Check sheet for the drawn part. Datum: minimum x, y, z corner. Units: mm. A direction names the side the tool comes from. Coordinates: 2 decimals unless noted, no trailing zeros. Write each loop counter-clockwise with the first axis right and the second up, starting at its lowest first coordinate (ties: lowest second). Pieces come first, ordered by that corner, then holes. Notation, with made-up numbers: (40.25, -14) -> (65.25, -14) arc R20 cw to (65.25, -10) -> close; hole circle Ø10 at (63.25, 80). An arc over 180 degrees is marked (long way). Answer in a Markdown table with one row per item.
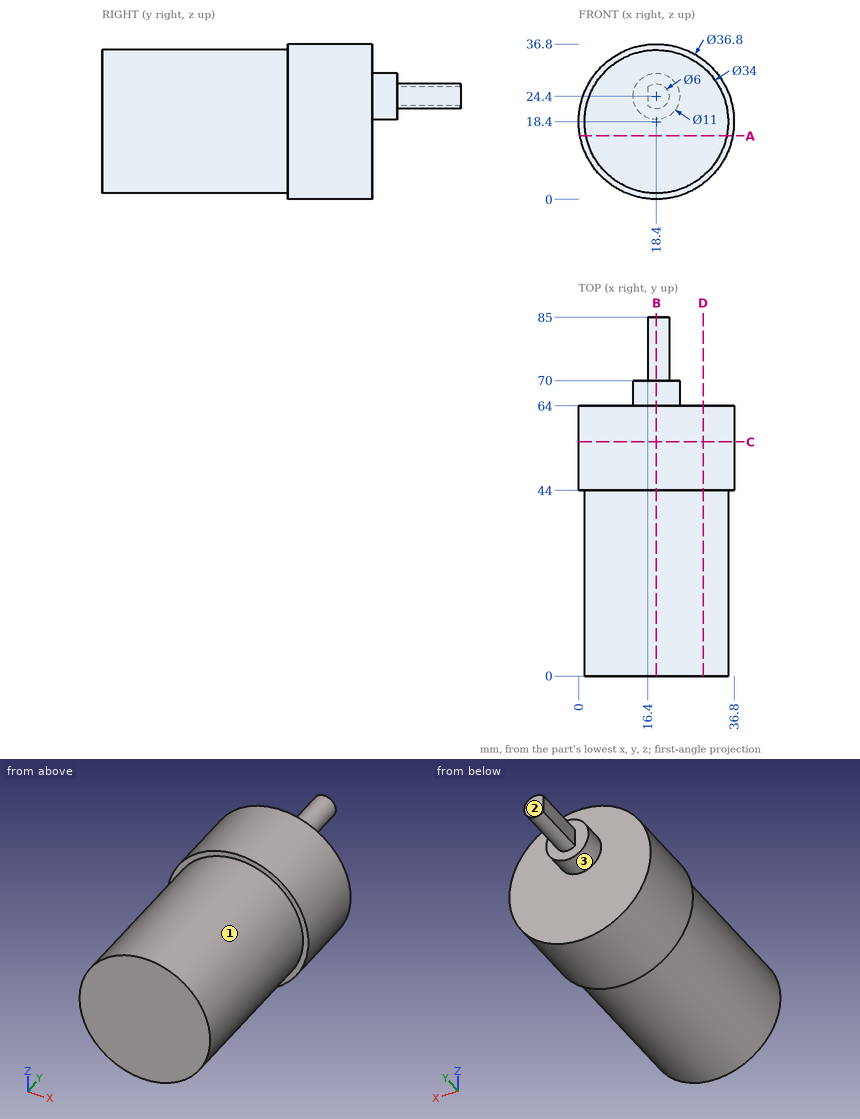
1. Sectioned sample at B-B, the plane x = 18.4. Record the cut outline in (y, z), and give its area (3 significant figures).
Findings below:
| item | result |
|---|---|
| outline | (0, 1.4) -> (44, 1.4) -> (44, 0) -> (64, 0) -> (64, 18.9) -> (70, 18.9) -> (70, 21.4) -> (85, 21.4) -> (85, 27.4) -> (70, 27.4) -> (70, 29.9) -> (64, 29.9) -> (64, 36.8) -> (44, 36.8) -> (44, 35.4) -> (0, 35.4) -> close |
| area | 2,390 mm² |
2. Sectioned sample at A-A, the plane z = 15. Record the cut outline in (x, y).
Findings below:
| item | result |
|---|---|
| outline | (0.32, 44) -> (1.74, 44) -> (1.74, 0) -> (35.06, 0) -> (35.06, 44) -> (36.48, 44) -> (36.48, 64) -> (0.32, 64) -> close |
3. Material ranges on probe 1 along Y at (x, z) = (25, 25.5); probe 2 along Y at (x, z) = (6.5, 32); probe 3 along X at (y, z) = (12, 19), recorded low to high. Write a range as from..to.
Findings below:
| item | result |
|---|---|
| probe 1 | y = 0..64 |
| probe 2 | y = 44..64 |
| probe 3 | x = 1.41..35.39 |
4. Sectioned sample at D-D, the plane x = 29.5. Record the cut outline in (y, z).
Findings below:
| item | result |
|---|---|
| outline | (0, 5.52) -> (44, 5.52) -> (44, 3.73) -> (64, 3.73) -> (64, 33.07) -> (44, 33.07) -> (44, 31.28) -> (0, 31.28) -> close |
5. Go/stop test with flat-tipped pins: pin 1 (12 mm diameter, centred on x = 29, y = 17, fed in from +Z); pin 2 (2 mm diameter, centred on x = 21.5, y = 30, fed in from -Z); pin 3 (4 mm diameter, centred on x = 8, y = 9.5, fed in from -Z). Record where each tip stops, or that it passes through.
Findings below:
| item | result |
|---|---|
| pin 1 | stops at z = 34.77 |
| pin 2 | stops at z = 1.53 |
| pin 3 | stops at z = 3.62 |
6. Access from +Z, -Z, +X, -X, +Y, -Y to the whole of each face (thin tool, end or side, straight path). Record for the marked faces 1, 2 and 3.
Findings below:
| item | result |
|---|---|
| face 1 | -Y |
| face 2 | +Z, -Z, +X, -X, +Y |
| face 3 | +Y |
7. Sectioned sample at C-C, the plane y = 55.5. Record the cut outline in (x, z).
Findings below:
| item | result |
|---|---|
| outline | circle Ø36.8 at (18.4, 18.4) |
